Check sheet for the modelled part. Datum: model origin and axes. Units: mm. Face numbers are marked on the shaded views. A direction names the side the tool comes from. Coordinates: 2 decimals unless noted, no trailing zeros. Write each loop counter-clockwise with the first axis right and the second up, starting at its lowest first coordinate (ties: lowest second). Pieces come first, ordered by that corner, then holes. Notation, with made-up numbers: (17.5, 49) -> (30.5, 49) arc R22 ccw to (30.5, 55) -> close; hole circle Ø9 at (71.5, 41). An arc over 180 degrees is marked (long way). Put each result on its own line as item: value.
```python
from build123d import *

# Parameters (mm, degrees)
SKETCH1_W                = 12.7
SKETCH1_H                = 17
BOSS_EXTRUDE1_DEPTH      = 1.5875
SKETCH2_W                = 1.5875
SKETCH2_H                = 17
BOSS_EXTRUDE2_DEPTH      = 11.1125
FILLET1_R                = 1
M2_CLEARANCE_HOLE1_D     = 2.4
M2_CLEARANCE_HOLE1_DEPTH = 2
M2_CLEARANCE_HOLE1_TIP   = 0.721032743
M2_CLEARANCE_HOLE2_D     = 2.4
M2_CLEARANCE_HOLE2_DEPTH = 2
M2_CLEARANCE_HOLE2_TIP   = 0.721032743


with BuildPart() as part:
    # Sketch1 → Boss-Extrude1 (new body)
    with BuildSketch(Plane(origin=(0, 0, 0), x_dir=(1, 0, 0), z_dir=(0, 1, 0))):
        with Locations((6.35, -8.5)):
            Rectangle(SKETCH1_W, SKETCH1_H)
    extrude(amount=BOSS_EXTRUDE1_DEPTH)

    # Sketch2 → Boss-Extrude2 (add)
    with BuildSketch(Plane(origin=(0, 1.5875, 0), x_dir=(1, 0, 0), z_dir=(0, 1, 0))):
        with Locations((0.79375, -8.5)):
            Rectangle(SKETCH2_W, SKETCH2_H)
    extrude(amount=BOSS_EXTRUDE2_DEPTH)

    # Fillet1
    fillet1_edges = [part.edges().sort_by_distance(p)[0] for p in [
        (0, 0, 8.5),
    ]]
    fillet(fillet1_edges, radius=FILLET1_R)

    # M2 Clearance Hole1
    with Locations(Plane(origin=(0, 0, 0), x_dir=(-1, 0, 0), z_dir=(0, -1, 0))):
        with Locations((-6.85, -8.5)):
            Hole(M2_CLEARANCE_HOLE1_D / 2, depth=M2_CLEARANCE_HOLE1_DEPTH)
            with Locations((0, 0, -(M2_CLEARANCE_HOLE1_DEPTH + M2_CLEARANCE_HOLE1_TIP / 2))):  # 118° drill point
                Cone(0, M2_CLEARANCE_HOLE1_D / 2, M2_CLEARANCE_HOLE1_TIP, mode=Mode.SUBTRACT)

    # M2 Clearance Hole2
    with Locations(Plane.ZY):
        with Locations((8.5, 6.85)):
            Hole(M2_CLEARANCE_HOLE2_D / 2, depth=M2_CLEARANCE_HOLE2_DEPTH)
            with Locations((0, 0, -(M2_CLEARANCE_HOLE2_DEPTH + M2_CLEARANCE_HOLE2_TIP / 2))):  # 118° drill point
                Cone(0, M2_CLEARANCE_HOLE2_D / 2, M2_CLEARANCE_HOLE2_TIP, mode=Mode.SUBTRACT)


solid = part.part
```
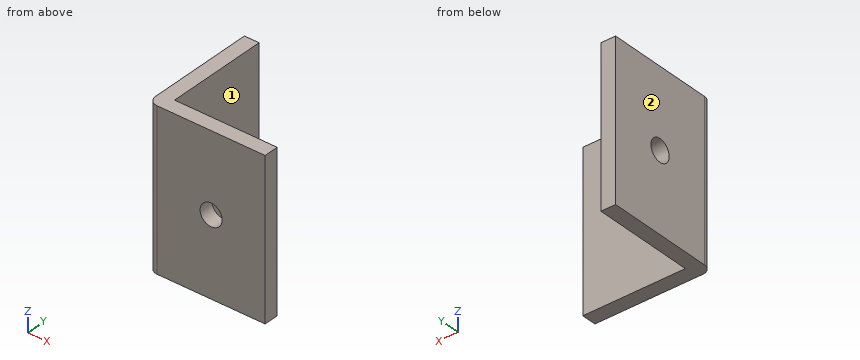
Q1. Cross-section at A-A (y = 6.85). Record the cut outline in (x, z), plus the area to 3 significant figures.
Recorded:
outline: (0, 0) -> (1.59, 0) -> (1.59, 7.3) -> (0, 7.3) -> close; (0, 9.7) -> (1.59, 9.7) -> (1.59, 17) -> (0, 17) -> close
area: 23.2 mm2
Q2. Cross-section at D-D (z = 15). Record the cut outline in (x, y).
Recorded:
outline: (0, 1) arc R1 ccw to (1, 0) -> (12.7, 0) -> (12.7, 1.59) -> (1.59, 1.59) -> (1.59, 12.7) -> (0, 12.7) -> close
Q3. Tool access check on the marked faces 1 and 2. Record the directions out of +Z, -Z, +X, -X, +Y, -Y that give a thin tool (end or side, any length) a straight path to the whole face; none if there is none.
Recorded:
face 1: +Z, -Z, +X, +Y
face 2: +Z, -Z, -X, +Y, -Y
Q4. Cross-section at C-C (z = 8.5). Record the cut outline in (x, y), plus the area to 3 significant figures.
Recorded:
outline: (0, 1) arc R1 ccw to (1, 0) -> (5.65, 0) -> (5.65, 1.59) -> (1.59, 1.59) -> (1.59, 5.65) -> (0, 5.65) -> close; (0, 8.05) -> (1.59, 8.05) -> (1.59, 12.7) -> (0, 12.7) -> close; (8.05, 0) -> (12.7, 0) -> (12.7, 1.59) -> (8.05, 1.59) -> close
area: 30.0 mm2
Q5. Material ranges on line 1 along Y through (x, z) = (0.95, 8.5); line 2 along Z through (x, y) = (6.85, 1), recorded low to high.
Recorded:
line 1: y = 0 to 5.65, 8.05 to 12.7
line 2: z = 0 to 7.3, 9.7 to 17
Q6. Depth check by flat-ended pin: P1, Ø3, axis at x = 4, z = 7, coming from the +Y side; P2, Ø5.5, axis at y = 5.5, z = 5.5, coming from the +X side. Enter the tip coordinate at first touch or a pass-through.
Recorded:
P1: stops at y = 1.59
P2: stops at x = 1.59
